from build123d import *

# Parameters (mm, degrees)
F0_W     = 97
F0_H     = 5
F0_R     = 1
F1_DEPTH = 10
F2_R     = 2.49999
F3_SIZE  = 1


# Not quite as in the source:
# - a fillet or chamfer is up to 0.001 mm smaller than in the source, because OpenCascade refuses the exact size


with BuildPart() as f1:
    # F0 (on Top) → F1 (new body)
    with BuildSketch(Plane.XY):
        Rectangle(F0_W, F0_H)
        with Locations((-46, 0)):
            Circle(F0_R, mode=Mode.SUBTRACT)
        with Locations((46, 0)):
            Circle(F0_R, mode=Mode.SUBTRACT)
    extrude(amount=F1_DEPTH)

    # F2 (radius 2.5 in the source; OpenCascade refuses exactly that, so slightly less here)
    f2_edges = [f1.edges().sort_by_distance(p)[0] for p in [
        (48.5, 2.5, 5),
        (48.5, -2.5, 5),
        (-48.5, 2.5, 5),
        (-48.5, -2.5, 5),
    ]]
    fillet(f2_edges, radius=F2_R)

    # F3
    f3_edges = [f1.edges().sort_by_distance(p)[0] for p in [
        (-47, 0, 10),
        (45, 0, 10),
        (45, 0, 0),
        (-47, 0, 0),
    ]]
    chamfer(f3_edges, length=F3_SIZE)


solid = f1.part
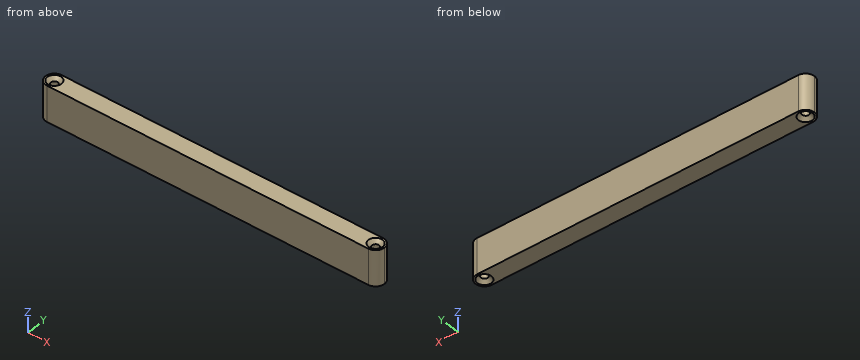
Design review of the part built by this model. Coordinates are the model's own, in mm. Round coordinates to 2 decimals unless told otherwise and drop trailing zeros. Answer as CSV lines item,"result". Start each with the question number.
1) Add section A-A (z = 4.5). Give the number of separate pieces and of enclosed holes in the cut face, then the cut area to 3 significant figures.
2) Wall thickness on line 1 along X through (y, z) = (0.35, 2.75); line 2 along Y through (x, z) = (46, 6); line 3 along X through (y, z) = (0.5, 2.25): over which ranges is each line inside the solid? List them lowest first. Write a range as [from, to].
3) For pin 1 Ø2.5 at (x, y) = (46, 0) entering from +Z; pin 2 Ø2.5 at (x, y) = (-46, 0) entering from -Z; pin 3 Ø1 at (y, z) = (1, 3.5) entering from +X, all flat-tipped, find the tip position at first contact; note any pin that passes through.
Resolved:
1,separate pieces,"1"
1,enclosed holes,"2"
1,area,"473 mm^2"
2,line 1,"[-48.48, -46.94], [-45.06, 45.06], [46.94, 48.48]"
2,line 2,"[-2.5, -1], [1, 2.5]"
2,line 3,"[-48.45, -46.87], [-45.13, 45.13], [46.87, 48.45]"
3,pin 1,"z = 9.25"
3,pin 2,"z = 0.75"
3,pin 3,"x = 48.45"
